```python
from build123d import *

# Parameters (mm, degrees)
F0_R     = 4.875428
F0_W     = 35
F0_H     = 12
F1_DEPTH = 3
F2_W     = 3.357807
F2_H     = 1.678903
F2_W_2   = 3.745247
F2_H_2   = 2.324635
F3_DEPTH = 5


with BuildPart() as f1:
    # F0 (on Top) → F1 (new body)
    with BuildSketch(Plane.XY):
        Polygon((-42.125307, -6), (-17.5, -6), (-17.5, 6), (-17.5, 11.001155), (-42.125307, 11.001155), align=None)
        with Locations((-35.409693, 0)):
            Circle(F0_R, mode=Mode.SUBTRACT)
        Rectangle(F0_W, F0_H)
    extrude(amount=F1_DEPTH)

    # F2 (on Right) → F3 (cut)
    with BuildSketch(Plane.YZ):
        with Locations((7.550389, 2.522841)):
            Rectangle(F2_W, F2_H)
        with Locations((-2.587604, 2.522841)):
            Rectangle(F2_W_2, F2_H_2)
    extrude(amount=-F3_DEPTH, mode=Mode.SUBTRACT)


solid = f1.part
```
Geometry check sheet. Reference: the model listing, model coordinates, mm. A direction names the side the tool comes from. Coordinates: 2 decimals unless noted, no trailing zeros. Loops run counter-clockwise (first coordinate to the right, second up) from the corner with the lowest first, then second, coordinate; pieces in that order, holes last. Notation, with made-up numbers: (-23, 85.25) - (14, 85.25) arc R25 ccw to (14, 104.25) - close; hole circle Ø8 at (3, -1). An arc over 180 degrees is marked (long way). One line per item, written item: value. Start each with the question number.
(1) Cross-section at B-B on x = -4.5. Enter the section's corners in (y, z).
(2) Cross-section at A-A on y = 0. Enter the section's corners in (x, z), plus the area to 3 significant figures.
(3) Cross-section at C-C on z = 0.6. Enter the section's corners in (x, y).
(4) Depth check by flat-ended pin: P1, Ø0.9, axis at y = 9.5, z = 1.5, coming from the +X side; P2, Ø1.1, axis at x = -3.5, y = -2.5, coming from the +Z side; P3, Ø0.5, axis at x = -2.5, z = 2.5, coming from the +Y side; P4, Ø6, axis at x = -35.41, y = 0, coming from the -Z side. Enter the tip coordinate at first touch or a pass-through.
(5) Material ranges on line 1 (X direction, y = -1, z = 1.5); line 2 (X direction, y = 9.5, z = 2.4); line 3 (X direction, y = 2.75, z = 2.05), recorded low to high. Write a range as [from, to].
(6) Cross-section at D-D on y = -3. Enter the section's corners in (x, z).
(7) Mould release check, pull along Y, two halves, no side actions. Record for faces 5 (the flat face through (-2, -0.715, 2)), 6 (the flat face through (0, 6, 1)), 7 (the flat face through (-13, -6, 1)), 8 (the flat face through (-2, -3, 1.361)): released by +Y, released by -Y, zero draft, split by the parting line, or undercut.
(8) Tool access check on faces 1 (the flat face through (-13, 1, 0)), 2 (the flat face through (-2, 5.871, 2)), 3 (the flat face through (-17.5, 8, 1)), 4 (the flat face through (-5, -3, 2)). Record the directions out of +Z, -Z, +X, -X, +Y, -Y that give a thin tool (end or side, any length) a straight path to the whole face; none if there is none.
Results below:
1. outline: (-6, 0) - (6, 0) - (6, 1.68) - (5.87, 1.68) - (5.87, 3) - (-0.71, 3) - (-0.71, 1.36) - (-4.46, 1.36) - (-4.46, 3) - (-6, 3) - close
2. outline: (-42.13, 0) - (-40.29, 0) - (-40.29, 3) - (-42.13, 3) - close; (-30.53, 0) - (17.5, 0) - (17.5, 3) - (-30.53, 3) - close
2. area: 150 mm2
3. outline: (-42.13, -6) - (17.5, -6) - (17.5, 6) - (-17.5, 6) - (-17.5, 11) - (-42.13, 11) - close; hole circle Ø9.75 at (-35.41, 0)
4. P1: stops at x = -17.5
4. P2: stops at z = 1.36
4. P3: stops at y = 5.87
4. P4: passes through
5. line 1: x = [-42.13, -40.18], [-30.64, -5], [0, 17.5]
5. line 2: x = [-42.13, -17.5]
5. line 3: x = [-42.13, -39.44], [-31.38, 17.5]
6. outline: (-42.13, 0) - (-39.25, 0) - (-39.25, 3) - (-42.13, 3) - close; (-31.57, 0) - (17.5, 0) - (17.5, 3) - (0, 3) - (0, 1.36) - (-5, 1.36) - (-5, 3) - (-31.57, 3) - close
7. face 5: undercut
7. face 6: released by +Y
7. face 7: released by -Y
7. face 8: undercut
8. face 1: -Z, +X, -X, +Y, -Y
8. face 2: +Z, +Y
8. face 3: +Z, -Z, +X, +Y
8. face 4: +Z
